Geometry: final body of the model. Coordinates: model frame, mm. Face numbers are marked on the shaded views. Give positions to 0.01 mm unless a question says otherwise; leave off trailing zeros. Write each loop counter-clockwise with the first axis right and the second up, starting at its lowest first coordinate (ties: lowest second). Pieces come first, ordered by that corner, then holes. Notation, with made-up numbers: M -17,24.25 L 37,24.25 A14 ccw 37,29.25 Z; hole C -36,84 d4. An arc over 180 degrees is marked long. One line per question, with ' | ' between items.
from build123d import *

# Parameters (mm, degrees)
SKETCH1_R           = 59.5
SKETCH1_R_2         = 52
BOSS_EXTRUDE1_DEPTH = 3.5
SKETCH2_R           = 61.75
BOSS_EXTRUDE2_DEPTH = 4
SKETCH3_R           = 59.5
SKETCH3_R_2         = 56
BOSS_EXTRUDE3_DEPTH = 2.5
FILLET1_R           = 2.5
SKETCH4_R           = 20
CUT_EXTRUDE1_DEPTH  = 22.5


with BuildPart() as part:
    # Sketch1 → Boss-Extrude1 (new body)
    with BuildSketch(Plane.XY):
        Circle(SKETCH1_R)
        Circle(SKETCH1_R_2, mode=Mode.SUBTRACT)
    extrude(amount=BOSS_EXTRUDE1_DEPTH)

    # Sketch2 → Boss-Extrude2 (add)
    with BuildSketch(Plane.XY.offset(3.5)):
        Circle(SKETCH2_R)
    extrude(amount=BOSS_EXTRUDE2_DEPTH)

    # Sketch3 → Boss-Extrude3 (add)
    with BuildSketch(Plane.XY.offset(7.5)):
        Circle(SKETCH3_R)
        Circle(SKETCH3_R_2, mode=Mode.SUBTRACT)
    extrude(amount=BOSS_EXTRUDE3_DEPTH)

    # Fillet1
    fillet1_edges = [part.edges().sort_by_distance(p)[0] for p in [
        (-56, 0, 10),
    ]]
    fillet(fillet1_edges, radius=FILLET1_R - 0.0001)  # a hair under: the kernel refuses the full size

    # Sketch4 → Cut-Extrude1 (cut)
    with BuildSketch(Plane.XY.offset(7.5)):
        Circle(SKETCH4_R)
    extrude(amount=-CUT_EXTRUDE1_DEPTH, mode=Mode.SUBTRACT)


solid = part.part
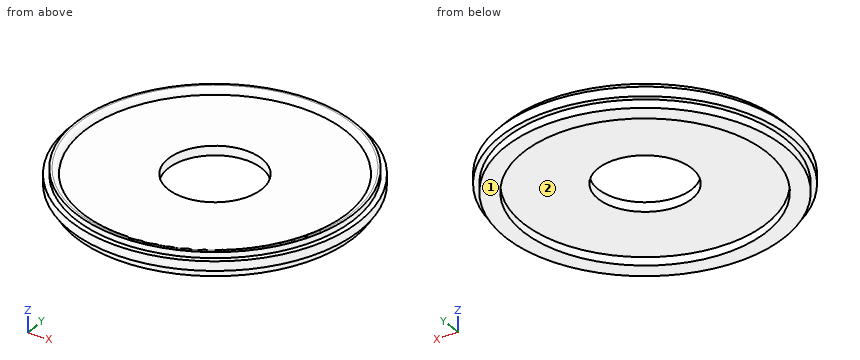
(1) Draft query along X for the marked faces 1 and 2. Return one class per face: released by +X, released by -X, zero draft, split by the parting line, or undercut.
Working result:
face 1: zero draft | face 2: undercut
(2) First-contact query: P1, Ø6, axis at x = -22, z = 3.5, coming from the -Y side; P2, Ø2, axis at y = -21.5, z = 1.5, coming from the -X side; P3, Ø1, axis at y = 31.5, z = 6.5, coming from the -X side. Flat tips, straight axial feed; report the tip coordinate or a pass-through.
Working result:
P1: stops at y = -58.75 | P2: stops at x = -55.86 | P3: stops at x = -53.4
(3) Cut plane C-C, the plane z = 1.5. Return loops of the section in (x, y).
Working result:
outline: C 0,0 d119; hole C 0,0 d104
(4) Material intervals for L1, parallel to Y at x = 0, z = 1.05; L2, parallel to Y at x = 0, z = 6.7; L3, parallel to Z at x = -39, y = 1, sorted ascending. Write a range as [from, to].
Working result:
L1: y = [-59.5, -52], [52, 59.5] | L2: y = [-61.75, -20], [20, 61.75] | L3: z = [3.5, 7.5]
